The listing builds one solid part. Answer for the finished solid, in the listing's coordinates (mm). Face numbers are marked on the shaded views. A direction names the side the tool comes from. Coordinates: 2 decimals unless noted, no trailing zeros. Write each loop counter-clockwise with the first axis right and the second up, starting at its lowest first coordinate (ties: lowest second). Pieces come first, ordered by that corner, then holes. Notation, with made-up numbers: M 63.5,20.5 L 93.5,20.5 A12 ccw 93.5,25.5 Z; hole C -16.5,-12.5 d10. An arc over 180 degrees is marked long. Put each result on its own line as item: value. Start each with the question number.
Autodesk Inventor part; units mm, degrees
ref_plane "Work Plane1" through (1.525, 0, 0) normal (0, 0, 1) x (1, 0, 0)
ref_plane "YZ Plane" through (0, 0, 0) normal (1, 0, 0) x (0, 1, 0)
ref_plane "XZ Plane" through (0, 0, 0) normal (0, 1, 0) x (-1, 0, 0)
sketch "Sketch1" plane through (0, 0, 0) normal (0, 0, 1) x (1, 0, 0)
  line L0 (0, 5) -> (0, 3)
  line L1 (3, 3) -> (16, 3)
  line L2 (16, 3) -> (16, 0)
  line L3 (16, 0) -> (-0.5001, 0)
  line L4 (-3.8001, 0) -> (19.3, 0)
  line L5 (-0.5001, 0) -> (-0.5001, 5)
  line L6 (-0.5001, 5) -> (0, 5)
  line L7 (3, 3) -> (2.3865, 3)
  line L8 (2.3865, 3) -> (0, 3)
  line L9 (0, -1) -> (0, 6)
  dimension "d0" = 16
  dimension "d1" = 13
  dimension "d2" = 6
  dimension "d9" = 0.5001
  dimension "d10" = 10
  dimension "d13" = 0.6136
  dimension "d14" = 6
revolve "Body" add sketch "Sketch1" angle 360 about axis through (16, 0, 0) along (-1, 0, 0)
sketch "Sketch2" plane through (-0.5001, 0, 0) normal (-1, 0, 0) x (0, 0, 1)
  line L0 (0, 5.7735) -> (5, 2.8868)
  line L1 (5, 2.8868) -> (5, -2.8868)
  line L2 (5, -2.8868) -> (0, -5.7735)
  line L3 (0, -5.7735) -> (-5, -2.8868)
  line L4 (-5, -2.8868) -> (-5, 2.8868)
  line L5 (-5, 2.8868) -> (0, 5.7735)
  point P0 (0, 0)
  point P1 (0, 0)
  dimension "d11" = 10
extrude "Head" add sketch "Sketch2" along normal blind 3.5
sketch "Sketch4" plane through (0, 0, 0) normal (0, 0, 1) x (1, 0, 0)
  line L0 (-4.0001, 5) -> (-4.0001, 5.7735)
  line L1 (-4.0001, 5.7735) -> (-3.5535, 5.7735)
  line L2 (-3.5535, 5.7735) -> (-4.0001, 5)
  line L3 (-4.7001, 0) -> (0.1999, 0)
  line L4 (-0.5001, 5.7735) -> (-4.0001, 5.7735)
  line L5 (-4.0001, 2.8868) -> (-4.0001, 5.7735)
  dimension "d5" = 30
  dimension "d19" = 10
revolve "Chamfer1" cut sketch "Sketch4" angle 360 about axis through (-10, 0, 0) along (1, 0, 0)
thread "Thread"
chamfer "Chamfer2" distance 0.6135 distance2 0.6136 1 edges at (16, -3, 0) measured on face at (16, -0.301, 1.1526)
ref_plane "Work Plane1" through (1.525, 0, 0) normal (0, 0, 1) x (1, 0, 0)
equation "\"d0\" = NLG"
equation "\"d1\" = GEL"
equation "\"d2\" = GD"
equation "\"d10\" = SD2"
equation "\"d14\" = BDM"
equation "\"d11\" = SW"
equation "\"d3\" = KOH - SD"
equation "\"d5\" = ANG1"
equation "\"d19\" = SW0"
equation "\"d15\" = GEL"
equation "\"d6\" = -0.5 * SPD + 0.5 * GD"
equation "\"NLG\" = 16"
equation "\"GD\" = NND"
equation "\"BDM\" = NND"
equation "\"KOH\" = 4"
equation "\"GEL\" = 13"
equation "\"SW\" = 10"
equation "\"SW0\" = SW"
equation "\"SPD\" = NND - 1.2269 * PTC"
equation "\"SD2\" = SW"
equation "\"SD\" = 0.5"
equation "\"ANG1\" = 30deg"
equation "\"GAL\" = 0.61345 * PTC"
equation "\"GUL\" = 0.61345 * PTC"
equation "\"RR\" = 0.25"
equation "\"WFT\" = SD"
equation "\"GD1\" = THREADDIA - 1.2269 * PTC"
equation "\"THREADDIA\" = 6"
equation "\"TOA\" = 30deg"
equation "\"FAWI\" = 45deg"
equation "\"PTC\" = 1"
equation "\"NND\" = 6"
equation "\"E0\" = 1.155 * SW"
properties part number "AS 1110 - M6 x 16" material "Steel, Mild"
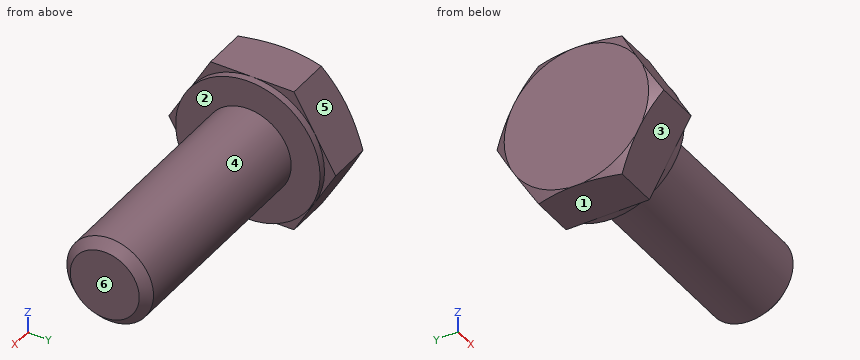
1) Determine the mould class of the marked faces 3, 4, 5 and 6 for opening direction Z: +Z half, -Z half, draft (parallel to the pull), parting line (faces both ways), or undercut.
2) Given pin 1 Ø2 at (y, z) = (-1.5, -4) entering from +X; pin 2 Ø1.5 at (x, y) = (11.5, -2.5) entering from -Z; pin 3 Ø0.7 at (y, z) = (5.5, 0.5) entering from +X, each flat-ended and moving along its own axis, determine where each tip first touches the part or whether it passes through.
3) A cutting plane is placed at A-A on x = 10.5. Write down the section's boundary in (y, z), then the cut area to 3 significant figures.
4) Straight lines are drawn through the part: probe 1 along X at (y, z) = (-3, 2); probe 2 along Y at (x, z) = (3.25, 0); probe 3 along Y at (x, z) = (6.75, -1.5). For each, find the intervals that lie inside material, in ascending order.
5) For the marked faces 1 and 2, determine the directions among +Z, -Z, +X, -X, +Y, -Y from which every point of the face is accessible in a straight line to the end or side of a thin tool.
Answers follow:
1. face 3: -Z half
1. face 4: parting line
1. face 5: +Z half
1. face 6: draft
2. pin 1: stops at x = 0
2. pin 2: stops at z = -2.44
2. pin 3: stops at x = -0.5
3. outline: C 0,0 d6
3. area: 28.3 mm²
4. probe 1: x = -4 to 0
4. probe 2: y = -3 to 3
4. probe 3: y = -2.6 to 2.6
5. face 1: -Z, +X, -X, +Y, -Y
5. face 2: +X
